Could you check a few things on this model? Use its own coordinates, in mm. Face numbers are marked on the shaded views. A direction names the side the tool comes from. Give positions to 0.01 mm unless a question says otherwise; leave off trailing zeros. Write each loop counter-clockwise with the first axis right and the second up, starting at its lowest first coordinate (ties: lowest second). Pieces come first, ordered by that corner, then holes. Notation, with made-up numbers: (11.5, 23) - (20.5, 23) arc R14 ccw to (20.5, 37) - close; hole circle Ø7 at (76.5, 51). An arc over 180 degrees is marked (long way). Answer as a JSON object with one key per item and string values. Group by question number.
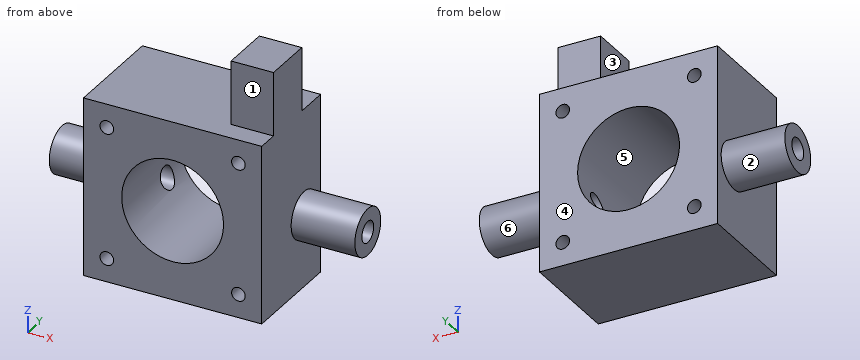
```python
from build123d import *

# Parameters (mm, degrees)
SKETCH_1_W           = 42
SKETCH_1_H           = 42
EXTRUDE_1_DEPTH      = 25
SKETCH_2_W           = 10
SKETCH_2_H           = 12
EXTRUDE_2_DEPTH      = 15
SKETCH_3_R           = 5.5
EXTRUDE_3_DEPTH      = 15
EXTRUDE_3_DEPTH_BACK = 57
CUT_EXTRUDE_1_REACH  = 74
SKETCH_4_R           = 2.5
CUT_EXTRUDE_2_REACH  = 27
SKETCH_5_R           = 12
SKETCH_5_R_2         = 1.6


with BuildPart() as part:
    # 草图1 → 凸台-拉伸1 (new body)
    with BuildSketch(Plane(origin=(0, 0, 0), x_dir=(1, 0, 0), z_dir=(0, 1, 0))):
        Rectangle(SKETCH_1_W, SKETCH_1_H)
    extrude(amount=EXTRUDE_1_DEPTH)

    # 草图2 → 凸台-拉伸2 (add)
    with BuildSketch(Plane.XY.offset(21)):
        with Locations((16, 11)):
            Rectangle(SKETCH_2_W, SKETCH_2_H)
    extrude(amount=EXTRUDE_2_DEPTH)

    # 草图3 → 凸台-拉伸3 (add, two sides)
    with BuildSketch(Plane(origin=(21, 0, 0), x_dir=(0, 0, -1), z_dir=(1, 0, 0))) as extrude_3_sk:
        with Locations((4, 18)):
            Circle(SKETCH_3_R)
    extrude(amount=EXTRUDE_3_DEPTH)
    extrude(extrude_3_sk.sketch, amount=-EXTRUDE_3_DEPTH_BACK)

    # 草图4 → 切除-拉伸1 (cut, up to next)
    with BuildSketch(Plane(origin=(36, 0, 0), x_dir=(0, 0, -1), z_dir=(1, 0, 0)), mode=Mode.PRIVATE) as cut_extrude_1_sk1:
        with Locations((4, 18)):
            Circle(SKETCH_4_R)
    cut_extrude_1_tool1 = extrude(cut_extrude_1_sk1.sketch, amount=-CUT_EXTRUDE_1_REACH, mode=Mode.PRIVATE) & part.part
    add(cut_extrude_1_tool1.solids().sort_by_distance((36, 18, -4))[0], mode=Mode.SUBTRACT)

    # 草图5 → 切除-拉伸2 (cut, up to next)
    with BuildSketch(Plane(origin=(0, 25, 0), x_dir=(1, 0, 0), z_dir=(0, 1, 0)), mode=Mode.PRIVATE) as cut_extrude_2_sk1:
        Circle(SKETCH_5_R)
    cut_extrude_2_tool1 = extrude(cut_extrude_2_sk1.sketch, amount=-CUT_EXTRUDE_2_REACH, mode=Mode.PRIVATE) & part.part
    add(cut_extrude_2_tool1.solids().sort_by_distance((0, 25, 0))[0], mode=Mode.SUBTRACT)
    # 草图5 → 切除-拉伸2 (cut, up to next)
    with BuildSketch(Plane(origin=(0, 25, 0), x_dir=(1, 0, 0), z_dir=(0, 1, 0)), mode=Mode.PRIVATE) as cut_extrude_2_sk2:
        with Locations((-15.5, 15.5)):
            Circle(SKETCH_5_R_2)
    cut_extrude_2_tool2 = extrude(cut_extrude_2_sk2.sketch, amount=-CUT_EXTRUDE_2_REACH, mode=Mode.PRIVATE) & part.part
    add(cut_extrude_2_tool2.solids().sort_by_distance((-15.5, 25, -15.5))[0], mode=Mode.SUBTRACT)
    # 草图5 → 切除-拉伸2 (cut, up to next)
    with BuildSketch(Plane(origin=(0, 25, 0), x_dir=(1, 0, 0), z_dir=(0, 1, 0)), mode=Mode.PRIVATE) as cut_extrude_2_sk3:
        with Locations((15.5, 15.5)):
            Circle(SKETCH_5_R_2)
    cut_extrude_2_tool3 = extrude(cut_extrude_2_sk3.sketch, amount=-CUT_EXTRUDE_2_REACH, mode=Mode.PRIVATE) & part.part
    add(cut_extrude_2_tool3.solids().sort_by_distance((15.5, 25, -15.5))[0], mode=Mode.SUBTRACT)
    # 草图5 → 切除-拉伸2 (cut, up to next)
    with BuildSketch(Plane(origin=(0, 25, 0), x_dir=(1, 0, 0), z_dir=(0, 1, 0)), mode=Mode.PRIVATE) as cut_extrude_2_sk4:
        with Locations((15.5, -15.5)):
            Circle(SKETCH_5_R_2)
    cut_extrude_2_tool4 = extrude(cut_extrude_2_sk4.sketch, amount=-CUT_EXTRUDE_2_REACH, mode=Mode.PRIVATE) & part.part
    add(cut_extrude_2_tool4.solids().sort_by_distance((15.5, 25, 15.5))[0], mode=Mode.SUBTRACT)
    # 草图5 → 切除-拉伸2 (cut, up to next)
    with BuildSketch(Plane(origin=(0, 25, 0), x_dir=(1, 0, 0), z_dir=(0, 1, 0)), mode=Mode.PRIVATE) as cut_extrude_2_sk5:
        with Locations((-15.5, -15.5)):
            Circle(SKETCH_5_R_2)
    cut_extrude_2_tool5 = extrude(cut_extrude_2_sk5.sketch, amount=-CUT_EXTRUDE_2_REACH, mode=Mode.PRIVATE) & part.part
    add(cut_extrude_2_tool5.solids().sort_by_distance((-15.5, 25, 15.5))[0], mode=Mode.SUBTRACT)


solid = part.part
```
(1) I need wall thicknesses on L1, parallel to Z at x = -15.5, y = 9; L2, parallel to Z at x = 15.5, y = 10. Which ranges of each line are inside material? Lowest first, please.
(2) For the marked faces 1, 2 and 3, which set-ups out of +Z, -Z, +X, -X, +Y, -Y let a thin tool reach every point of the face, with its end or its side?
(3) I want a section at A-A, the plane x = -15.5. Please give me the cut outline in (y, z).
(4) I want a section at D-D, the plane y = 18. Please give me the cut outline in (x, z).
(5) Will these pins go through, and if not, where does the flat tip stop? P1, Ø3, axis at x = 17, z = 29, coming from the -Y side; P2, Ø1.9, axis at x = -15.5, z = -15.5, coming from the -Y side; P3, Ø6, axis at y = 18.5, z = 11.5, coming from the +X side; P4, Ø2, axis at y = 12, z = -8, coming from the -X side.
(6) I want a section at B-B, the plane z = 15.5. Please give me the cut outline in (x, y).
(7) I want a section at C-C, the plane x = 0. Please give me the cut outline in (y, z).
(8) If we mould it in two halves opening along Z, with no side actions, what happens to the marked faces 4, 5 and 6? For each: +Z half, -Z half, draft (parallel to the pull), parting line (faces both ways), or undercut.
Entries:
{
 "1": {"L1": "-21 to -17.1, -13.9 to 13.9, 17.1 to 21", "L2": "-21 to -17.1, -13.9 to 13.9, 17.1 to 36"},
 "2": {"face 1": "+Z, +X, -X, -Y", "face 2": "-X", "face 3": "+Z, -X, +Y, -Y"},
 "3": {"outline": "(0, -21) - (25, -21) - (25, -17.1) - (0, -17.1) - close; (0, -13.9) - (25, -13.9) - (25, 13.9) - (0, 13.9) - close; (0, 17.1) - (25, 17.1) - (25, 21) - (0, 21) - close; hole circle Ø5 at (18, -4)"},
 "4": {"outline": "(-36, -9.5) - (-21, -9.5) - (-21, -21) - (21, -21) - (21, -9.5) - (36, -9.5) - (36, -6.5) - (10.09, -6.5) arc R12 cw to (-10.09, -6.5) - (-36, -6.5) - close; (-36, -1.5) - (-11.91, -1.5) arc R12 cw (long way) to (11.91, -1.5) - (36, -1.5) - (36, 1.5) - (21, 1.5) - (21, 21) - (-21, 21) - (-21, 1.5) - (-36, 1.5) - close; hole circle Ø3.2 at (-15.5, -15.5); hole circle Ø3.2 at (-15.5, 15.5); hole circle Ø3.2 at (15.5, -15.5); hole circle Ø3.2 at (15.5, 15.5)"},
 "5": {"P1": "y = 5", "P2": "through", "P3": "x = 21", "P4": "x = -21"},
 "6": {"outline": "(-21, 0) - (-17.1, 0) - (-17.1, 25) - (-21, 25) - close; (-13.9, 0) - (13.9, 0) - (13.9, 25) - (-13.9, 25) - close; (17.1, 0) - (21, 0) - (21, 25) - (17.1, 25) - close"},
 "7": {"outline": "(0, -21) - (25, -21) - (25, -12) - (0, -12) - close; (0, 12) - (25, 12) - (25, 21) - (0, 21) - close"},
 "8": {"face 4": "draft", "face 5": "undercut", "face 6": "parting line"}
}
